Input: part model. Units: mm. Frame: model coordinates. Coordinates: 2 decimals unless noted, no trailing zeros. Loops run counter-clockwise (first coordinate to the right, second up) from the corner with the lowest first, then second, coordinate; pieces in that order, holes last.
Item 1: Section B-B on x = 193. Return loops of the section in (y, z).
Item 2: Contact query for a flat-ended pin moving along its axis: P1, Ø0.5, axis at x = 10, z = 0.5, coming from the +Y side. Output: stop coordinate, or through.
Item 3: Ray query, line 1 along X through (y, z) = (174, 0.7); line 2 along Y through (x, z) = (-144, 0.55); line 3 along Y through (x, z) = (191, 0.9). Return the intervals inside material, ascending.
Item 4: Section C-C on z = 0.7. Give the number of separate pieces and of enclosed holes in the cut face, and give its area (3 significant figures).
Item 5: Section D-D on x = 14. Return loops of the section in (y, z), and give its area (3 significant figures).
Item 6: Section A-A on y = 93. Return loops of the section in (x, z), and give its area (3 significant figures).
```python
from build123d import *

# Parameters (mm, degrees)
SKETCH_1_W          = 470
SKETCH_1_H          = 600
EXTRUDE_1_DEPTH     = 1
HOLE_WIZARD_M5_1_D  = 5.5
SKETCH_1_3_W        = 300
SKETCH_1_3_H        = 142
CUT_EXTRUDE_3_DEPTH = 10
SKETCH_4_W          = 30
SKETCH_4_H          = 60
CUT_EXTRUDE_4_DEPTH = 10
SKETCH_5_R          = 3
CUT_EXTRUDE_5_DEPTH = 10


with BuildPart() as part:
    # 스케치1 → 보스-돌출1 (new body)
    with BuildSketch(Plane.XY):
        Rectangle(SKETCH_1_W, SKETCH_1_H)
    extrude(amount=EXTRUDE_1_DEPTH)

    # M5 여유 구멍1 (through all)
    with Locations(Plane(origin=(0, 0, 0), x_dir=(-1, 0, 0), z_dir=(0, 0, -1))):
        with Locations((-225, 290), (-135, 290), (-45, 290), (45, 290), (135, 290), (225, 290), (225, 174), (225, 58), (225, -58), (225, -174), (225, -290), (-225, 174), (-225, 58), (-225, -58), (-225, -174), (-225, -290), (-135, -290), (-45, -290), (45, -290), (135, -290)):
            Hole(HOLE_WIZARD_M5_1_D / 2)

    # 스케치1<3> → 컷-돌출3 (cut)
    with BuildSketch(Plane.XY):
        with Locations((0, 229)):
            Rectangle(SKETCH_1_3_W, SKETCH_1_3_H)
    extrude(amount=CUT_EXTRUDE_3_DEPTH, mode=Mode.SUBTRACT)

    # 스케치4 → 컷-돌출4 (cut)
    with BuildSketch(Plane.XY.offset(1)):
        with Locations((192.5, 113)):
            Rectangle(SKETCH_4_W, SKETCH_4_H)
        with BuildLine():
            Line((-187.5, -105.5), (-47.5, -105.5))
            ThreePointArc((-47.5, -105.5), (-40.428932188, -108.428932188), (-37.5, -115.5))
            Line((-37.5, -115.5), (-37.5, -255.5))
            ThreePointArc((-37.5, -255.5), (-40.428932188, -262.571067812), (-47.5, -265.5))
            Line((-47.5, -265.5), (-187.5, -265.5))
            ThreePointArc((-187.5, -265.5), (-194.571067812, -262.571067812), (-197.5, -255.5))
            Line((-197.5, -255.5), (-197.5, -115.5))
            ThreePointArc((-197.5, -115.5), (-194.571067812, -108.428932188), (-187.5, -105.5))
        make_face()
    extrude(amount=-CUT_EXTRUDE_4_DEPTH, mode=Mode.SUBTRACT)

    # 스케치5 → 컷-돌출5 (cut)
    with BuildSketch(Plane.XY.offset(1)):
        with Locations((-171, -98.5)):
            Circle(SKETCH_5_R)
        with Locations((-144, -98.5)):
            Circle(SKETCH_5_R)
        with Locations((-91, -98.5)):
            Circle(SKETCH_5_R)
        with Locations((-64, -98.5)):
            Circle(SKETCH_5_R)
    extrude(amount=-CUT_EXTRUDE_5_DEPTH, mode=Mode.SUBTRACT)


solid = part.part
```
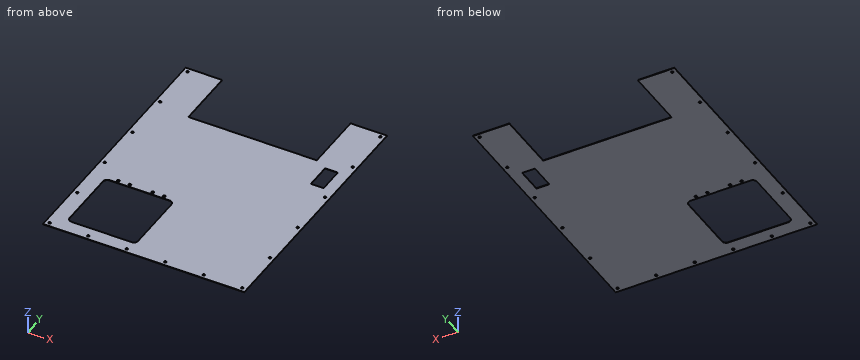
Results found:
1. outline: (-300, 0) - (83, 0) - (83, 1) - (-300, 1) - close; (143, 0) - (300, 0) - (300, 1) - (143, 1) - close
2. P1: stops at y = 158
3. line 1: x = -235 to -227.75, -222.25 to -150, 150 to 222.25, 227.75 to 235
3. line 2: y = -300 to -265.5, -105.5 to -101.5, -95.5 to 158
3. line 3: y = -300 to 83, 143 to 300
4. separate pieces: 1
4. enclosed holes: 22
4. area: 212,000 mm2
5. outline: (-300, 0) - (158, 0) - (158, 1) - (-300, 1) - close
5. area: 458 mm2
6. outline: (-235, 0) - (177.5, 0) - (177.5, 1) - (-235, 1) - close; (207.5, 0) - (235, 0) - (235, 1) - (207.5, 1) - close
6. area: 440 mm2
